CAD build for the part. Positions are in the model's coordinates, mm. Round coordinates to 2 decimals unless told otherwise and drop trailing zeros. Order: outer loops, then holes, each group sorted by start corner. A loop starts at its lowest first (then second) coordinate and runs counter-clockwise, first axis right, second up. Notation, with made-up numbers: (-36, -32.5) - (13, -32.5) arc R26 cw to (13, -6.5) - close; hole circle Ø7 at (26, 74). An arc over 180 degrees is marked (long way). Write item = value, one per line.
from build123d import *

# Parameters (mm, degrees)
F0_R     = 2.424029
F0_R_2   = 1.984375
F1_DEPTH = 3.175


with BuildPart() as f1:
    # F0 (on Right) → F1 (new body)
    with BuildSketch(Plane.YZ):
        Polygon((-101.6, -81.478684), (-50.8, -81.478684), (-50.8, -78.176684), (-25.4, -78.176684), (-25.4, -81.478684), (25.4, -81.478684), (25.4, -78.176684), (50.8, -78.176684), (50.8, -81.478684), (101.6, -81.478684), (101.6, -78.176684), (149.098, -78.176684), (149.098, -60.396684), (152.273, -60.396684), (152.273, -42.616684), (149.098, -42.616684), (149.098, -24.836684), (152.273, -24.836684), (152.273, -7.056684), (149.098, -7.056684), (149.098, 10.723316), (152.273, 10.723316), (152.273, 28.503316), (149.098, 28.503316), (149.098, 46.283316), (101.6, 46.283316), (101.6, 49.585316), (50.8, 49.585316), (50.8, 46.283316), (25.4, 46.283316), (25.4, 49.585316), (-25.4, 49.585316), (-25.4, 46.283316), (-50.8, 46.283316), (-50.8, 49.585316), (-101.6, 49.585316), (-101.6, 46.283316), (-149.098, 46.283316), (-149.098, 28.503316), (-152.273, 28.503316), (-152.273, 10.723316), (-149.098, 10.723316), (-149.098, -7.056684), (-152.273, -7.056684), (-152.273, -24.836684), (-149.098, -24.836684), (-149.098, -42.616684), (-152.273, -42.616684), (-152.273, -60.396684), (-149.098, -60.396684), (-149.098, -78.176684), (-101.6, -78.176684), align=None)
        with Locations((-139.573, -68.651684)):
            Circle(F0_R, mode=Mode.SUBTRACT)
        with Locations((-126.873, -68.651684)):
            Circle(F0_R, mode=Mode.SUBTRACT)
        with Locations((-139.573, -55.951684)):
            Circle(F0_R, mode=Mode.SUBTRACT)
        with Locations((-126.873, -55.951684)):
            Circle(F0_R, mode=Mode.SUBTRACT)
        with Locations((-88.9, -30.678684)):
            Circle(F0_R_2, mode=Mode.SUBTRACT)
        with Locations((-38.1, -30.678684)):
            Circle(F0_R_2, mode=Mode.SUBTRACT)
        with Locations((-25.4, -30.678684)):
            Circle(F0_R_2, mode=Mode.SUBTRACT)
        with Locations((-12.7, -30.678684)):
            Circle(F0_R_2, mode=Mode.SUBTRACT)
        with Locations((126.873, -68.651684)):
            Circle(F0_R, mode=Mode.SUBTRACT)
        with Locations((139.573, -68.651684)):
            Circle(F0_R, mode=Mode.SUBTRACT)
        with Locations((126.873, -55.951684)):
            Circle(F0_R, mode=Mode.SUBTRACT)
        with Locations((139.573, -55.951684)):
            Circle(F0_R, mode=Mode.SUBTRACT)
        with Locations((12.7, -30.678684)):
            Circle(F0_R_2, mode=Mode.SUBTRACT)
        with Locations((25.4, -30.678684)):
            Circle(F0_R_2, mode=Mode.SUBTRACT)
        with Locations((38.1, -30.678684)):
            Circle(F0_R_2, mode=Mode.SUBTRACT)
        with Locations((88.9, -30.678684)):
            Circle(F0_R_2, mode=Mode.SUBTRACT)
    extrude(amount=F1_DEPTH)


solid = f1.part
(1) Probe line 1 along Z through (x, y) = (1.45, 12.7); line 2 along Z through (x, y) = (1.65, -38.1); line 3 along Z through (x, y) = (1.3, -111). List the from-to ranges inside material, lowest first.
Solved:
line_1 = -81.48 to -32.66, -28.69 to 49.59
line_2 = -78.18 to -32.66, -28.69 to 46.28
line_3 = -78.18 to 46.28
(2) Drop flat-ended pins along their axis: pin 1 (1 mm diameter, centred on x = 1, y = 41.5, fed in from +Z); pin 2 (4.5 mm diameter, centred on y = 139.57, z = -68.65, fed in from +X); pin 3 (1 mm diameter, centred on x = 1, y = -150.5, fed in from +Z); pin 4 (1 mm diameter, centred on x = 1, y = -150.5, fed in from -Z). Give the stop position or say it passes through.
Solved:
pin_1 = 46.28
pin_2 = through
pin_3 = 28.5
pin_4 = -60.4
(3) Band-saw the part on A-A on z = 8. List the corners of the cut face in (x, y) (3 decimals).
Solved:
outline = (0, -149.098) - (3.175, -149.098) - (3.175, 149.098) - (0, 149.098) - close
(4) Band-saw the part on B-B on x = 1.55. Count the separate pieces of the cut face and the enclosed holes in it, plus the area to 3 significant figures.
Solved:
separate_pieces = 1
enclosed_holes = 16
area = 38,200 mm²
